```python
from build123d import *

# Parameters (mm, degrees)
F0_R         = 17.78
F0_W         = 50.8
F0_H         = 38.1
F0_R_2       = 7.62
F1_DEPTH     = 9.398
F2_W         = 12.4930366991
F2_H         = 2.54
F3_DEPTH     = 6.35
F4_W         = 9.7033483908
F4_H         = 2.4660443887
F4_R         = 1.3462908927
F4_R_2       = 1.087736237
F5_DEPTH     = 3.1496
F6_DEPTH     = 0.2286
F7_R         = 0.3066051224
F8_T1_DEPTH  = 93.98
F8_T3_DEPTH  = 50.8
F8_T6_ANGLE  = 90
F8_T8_ANGLE  = 90
F8_T10_ANGLE = 90
F8_T12_ANGLE = 90
F9_START     = 8.128
F9_DEPTH     = 1.524


# Not quite as in the source:
# - a fillet or chamfer that OpenCascade refuses, or shapes differently, is made with other operations: its cross-section is extruded or revolved along the edge and cut away or added


with BuildPart() as f1:
    # F0 (on Top) → F1 (new body)
    with BuildSketch(Plane.XY):
        with BuildLine():
            Line((25.4, 52.07), (-25.4, 52.07))
            ThreePointArc((-25.4, 52.07), (-28.9921024484, 50.5821024484), (-30.48, 46.99))
            Line((-30.48, 46.99), (-30.48, -46.99))
            ThreePointArc((-30.48, -46.99), (-28.9921024484, -50.5821024484), (-25.4, -52.07))
            Line((-25.4, -52.07), (25.4, -52.07))
            ThreePointArc((25.4, -52.07), (28.9921024484, -50.5821024484), (30.48, -46.99))
            Line((30.48, -46.99), (30.48, 46.99))
            ThreePointArc((30.48, 46.99), (28.9921024484, 50.5821024484), (25.4, 52.07))
        make_face()
        with Locations((0, -21.59)):
            Circle(F0_R, mode=Mode.SUBTRACT)
        with Locations((0, 27.94)):
            Rectangle(F0_W, F0_H, mode=Mode.SUBTRACT)
        with Locations((0, -21.59)):
            Circle(F0_R)
        with Locations((0, -21.59)):
            Circle(F0_R_2, mode=Mode.SUBTRACT)
        with Locations((0, -21.59)):
            Circle(F0_R_2)
        with Locations((0, 27.94)):
            Rectangle(F0_W, F0_H)
    extrude(amount=F1_DEPTH)

    # F2 (on face) → F3 (cut)
    with BuildSketch(Plane.XZ.offset(52.07)):
        with Locations((-0.0956295989, 3.81)):
            Rectangle(F2_W, F2_H)
    extrude(amount=-F3_DEPTH, mode=Mode.SUBTRACT)

    # F4 (on face) → F5 (cut)
    with BuildSketch(Plane(origin=(0, 52.07, 0), x_dir=(-1, 0, 0), z_dir=(0, 1, 0))):
        with Locations((-17.8750143386, 7.5830221944)):
            Rectangle(F4_W, F4_H)
        with Locations((18.9737091073, 7.7977091073)):
            Circle(F4_R)
        with Locations((18.9737091073, 7.7977091073)):
            Circle(F4_R_2, mode=Mode.SUBTRACT)
    extrude(amount=-F5_DEPTH, mode=Mode.SUBTRACT)

    # F6 (add): a face of the model
    f6_faces = [f1.faces().sort_by_distance(p)[0] for p in [
        (-18.9737091073, 52.07, 7.7977091073),
    ]]
    extrude(f6_faces, amount=F6_DEPTH)

    # F7
    f7_edges = [f1.edges().sort_by_distance(p)[0] for p in [
        (-17.885973, 52.2986, 7.797709),
    ]]
    fillet(f7_edges, radius=F7_R)

    # F8: fillet of radius 5.08 on 1 edges, made by hand

    # F8_s2 → F8_t1 (cut)
    with BuildSketch(Plane.XZ.offset(-46.99)):
        with BuildLine():
            ThreePointArc((-25.4, 0), (-28.9921024484, 1.4878975516), (-30.48, 5.08))
            Line((-30.48, 5.08), (-30.48, 0))
            Line((-30.48, 0), (-25.4, 0))
        make_face()
        with BuildLine():
            ThreePointArc((25.4, 0), (28.9921024484, 1.4878975516), (30.48, 5.08))
            Line((30.48, 5.08), (30.48, 0))
            Line((30.48, 0), (25.4, 0))
        make_face()
    extrude(amount=F8_T1_DEPTH, mode=Mode.SUBTRACT)

    # F8_s4 → F8_t3 (cut)
    with BuildSketch(Plane.YZ.offset(-25.4)):
        with BuildLine():
            ThreePointArc((-46.99, 0), (-50.5821024484, 1.4878975516), (-52.07, 5.08))
            Line((-52.07, 5.08), (-52.07, 0))
            Line((-52.07, 0), (-46.99, 0))
        make_face()
        with BuildLine():
            ThreePointArc((52.07, 5.08), (50.5821024484, 1.4878975516), (46.99, 0))
            Line((46.99, 0), (52.07, 0))
            Line((52.07, 0), (52.07, 5.08))
        make_face()
    extrude(amount=F8_T3_DEPTH, mode=Mode.SUBTRACT)

    # F8_s5 → F8_t6 (revolve, cut)
    with BuildSketch(Plane.XZ.offset(46.99)):
        with BuildLine():
            ThreePointArc((-25.4, 0), (-28.9921024484, 1.4878975516), (-30.48, 5.08))
            Line((-30.48, 5.08), (-30.48, 0))
            Line((-30.48, 0), (-25.4, 0))
        make_face()
    revolve(axis=Axis((-25.4, -46.99, 0), (0, 0, 1)), revolution_arc=F8_T6_ANGLE, mode=Mode.SUBTRACT)

    # F8_s7 → F8_t8 (revolve, cut)
    with BuildSketch(Plane.YZ.offset(25.4)):
        with BuildLine():
            ThreePointArc((-46.99, 0), (-50.5821024484, 1.4878975516), (-52.07, 5.08))
            Line((-52.07, 5.08), (-52.07, 0))
            Line((-52.07, 0), (-46.99, 0))
        make_face()
    revolve(axis=Axis((25.4, -46.99, 0), (0, 0, 1)), revolution_arc=F8_T8_ANGLE, mode=Mode.SUBTRACT)

    # F8_s9 → F8_t10 (revolve, cut)
    with BuildSketch(Plane.XZ.offset(-46.99)):
        with BuildLine():
            ThreePointArc((30.48, 5.08), (28.9921024484, 1.4878975516), (25.4, 0))
            Line((25.4, 0), (30.48, 0))
            Line((30.48, 0), (30.48, 5.08))
        make_face()
    revolve(axis=Axis((25.4, 46.99, 0), (0, 0, 1)), revolution_arc=F8_T10_ANGLE, mode=Mode.SUBTRACT)

    # F8_s11 → F8_t12 (revolve, cut)
    with BuildSketch(Plane.YZ.offset(-25.4)):
        with BuildLine():
            ThreePointArc((46.99, 0), (50.5821024484, 1.4878975516), (52.07, 5.08))
            Line((52.07, 5.08), (52.07, 0))
            Line((52.07, 0), (46.99, 0))
        make_face()
    revolve(axis=Axis((-25.4, 46.99, 0), (0, 0, 1)), revolution_arc=F8_T12_ANGLE, mode=Mode.SUBTRACT)

    # F0 (on Top) → F9 (cut)
    with BuildSketch(Plane.XY.offset(F9_START)):
        with Locations((0, 27.94)):
            Rectangle(F0_W, F0_H)
    extrude(amount=F9_DEPTH, mode=Mode.SUBTRACT)

    # F10 (on Right) → F11 (revolve, cut)
    with BuildSketch(Plane.YZ):
        Polygon((-7.623700425, 9.6026211977), (-22.3824381828, 9.6026211977), (-22.3824381828, 7.986061275), (-13.9484070241, 7.986061275), align=None)
    revolve(axis=Axis((0, -22.3824381828, 9.8022762686), (0, 0, 1)), mode=Mode.SUBTRACT)


solid = f1.part
```
The listing builds one solid part. Answer for the finished solid, in the listing's coordinates (mm). A direction names the side the tool comes from. Give positions to 0.01 mm unless a question says otherwise; leave off trailing zeros. Loops run counter-clockwise (first coordinate to the right, second up) from the corner with the lowest first, then second, coordinate; pieces in that order, holes last. Notation, with made-up numbers: M 49,-0.75 L 108,-0.75 A25 ccw 108,17.25 Z; hole C 39.5,50.5 d6. An arc over 180 degrees is marked long. One line per item, written item: value.
Q1. A cutting plane is placed at D-D on y = 44.5. Determine the outline of the cut face in (x, z).
Working result:
outline: M -30.48,5.08 A5.08 ccw -25.4,0 L 25.4,0 A5.08 ccw 30.48,5.08 L 30.48,9.4 L 25.4,9.4 L 25.4,8.13 L -25.4,8.13 L -25.4,9.4 L -30.48,9.4 Z
Q2. Determine the mould class of faces 1 (the face through (0, -22, 7.986)), 2 (the face through (-17.981, 50.517, 8.708)), 3 (the face through (-30.48, 1, 7)) for opening direction Z: +Z half, -Z half, draft (parallel to the pull), parting line (faces both ways), or undercut.
Working result:
face 1: +Z half
face 2: undercut
face 3: draft
Q3. A cutting plane is placed at A-A on x = 0. Determine the outline of the cut face in (y, z).
Working result:
outline: M -52.07,5.08 L -45.72,5.08 L -45.72,2.54 L -51.39,2.54 A5.08 ccw -46.99,0 L 46.99,0 A5.08 ccw 52.07,5.08 L 52.07,9.4 L 46.99,9.4 L 46.99,8.13 L 8.89,8.13 L 8.89,9.4 L -8.42,9.4 L -13.95,7.99 L -30.82,7.99 L -36.34,9.4 L -52.07,9.4 Z
Q4. For faces 4 (the face through (-6.342, -49, 4)), 5 (the face through (30.48, -1, 7)), 6 (the face through (18, 51, 8.816)), determine the directions among +Z, -Z, +X, -X, +Y, -Y from which every point of the face is accessible in a straight line to the end or side of a thin tool.
Working result:
face 4: -Y
face 5: +Z, -Z, +X, +Y, -Y
face 6: +Y
Q5. A cutting plane is placed at C-C on z = 1.5. Determine the outline of the cut face in (x, y), then the cut area to 3 significant figures.
Working result:
outline: M -29,-46.99 A3.6 ccw -25.4,-50.59 L 25.4,-50.59 A3.6 ccw 29,-46.99 L 29,46.99 A3.6 ccw 25.4,50.59 L -25.4,50.59 A3.6 ccw -29,46.99 Z
area: 5,860 mm^2
Q6. A cutting plane is placed at B-B on y = -5.5. Determine the outline of the cut face in (x, z).
Working result:
outline: M -30.48,5.08 A5.08 ccw -25.4,0 L 25.4,0 A5.08 ccw 30.48,5.08 L 30.48,9.4 L -30.48,9.4 Z
Q7. Flat-ended cylindrical pins translate along their axes: P1, Ø18.5, axis at x = 1, y = -24, coming from the +Z side; P2, Ø5, axis at y = -10.5, z = 1.5, coming from the -X side; P3, Ø1, axis at x = -1, z = 8, coming from the +Y side. Find the tip coordinate at first contact, or state that the pin passes through.
Working result:
P1: stops at z = 8.68
P2: stops at x = -30.36
P3: stops at y = 52.07
Q8. Find the intervals of material crossed by line 1 (Y direction, x = -22, z = 8.25); line 2 (Z direction, x = -1, y = -47); line 3 (Y direction, x = 9, z = 8), in increasing order. Write a range as from..to.
Working result:
line 1: y = -52.07..8.89, 46.99..52.07
line 2: z = 0..2.54, 5.08..9.4
line 3: y = -52.07..52.07
